Part model, mm, in its own coordinate system. A direction names the side the tool comes from. Give positions to 0.01 mm unless a question says otherwise; leave off trailing zeros. Write each loop counter-clockwise with the first axis right and the second up, starting at its lowest first coordinate (ties: lowest second). Pieces come first, ordered by that corner, then holes.
```python
from build123d import *

# Parameters (mm, degrees)
SALIENTE_EXTRUIR1_DEPTH      = 45
CORTAR_EXTRUIR1_DEPTH        = 35
CORTAR_EXTRUIR1_DEPTH_BACK   = 25
SALIENTE_EXTRUIR2_DEPTH      = 0.0001
SALIENTE_EXTRUIR2_DEPTH_BACK = 10
CORTAR_EXTRUIR2_DEPTH        = 50.0001
CROQUIS5_R                   = 2.5
CORTAR_EXTRUIR3_DEPTH        = 20
CROQUIS6_W                   = 35
CROQUIS6_H                   = 5
CORTAR_EXTRUIR4_DEPTH        = 50
REDONDEO7_R                  = 10
SALIENTE_EXTRUIR3_DEPTH      = 45


with BuildPart() as part:
    # Croquis1 → Saliente-Extruir1 (new body)
    with BuildSketch(Plane.XY):
        with BuildLine():
            Line((5.169872345, 17.452931937), (-42.830127655, 37.452931937))
            Line((-42.830127655, 37.452931937), (-42.830127655, 17.452931937))
            Line((-42.830127655, 17.452931937), (-34.437895384, -24.508229414))
            ThreePointArc((-34.437895384, -24.508229414), (-30.971977683, -30.280489476), (-24.632088627, -32.547068063))
            Line((-24.632088627, -32.547068063), (-22.830127655, -32.547068063))
            Line((-22.830127655, -32.547068063), (-22.830127655, -12.547068063))
            ThreePointArc((-22.830127655, -12.547068063), (-18.830127655, -8.547068063), (-14.830127655, -12.547068063))
            Line((-14.830127655, -12.547068063), (-14.830127655, -32.547068063))
            Line((-14.830127655, -32.547068063), (-13.028166682, -32.547068063))
            ThreePointArc((-13.028166682, -32.547068063), (-6.688277626, -30.280489476), (-3.222359925, -24.508229414))
            Line((-3.222359925, -24.508229414), (5.169872345, 17.452931937))
        make_face()
    extrude(amount=SALIENTE_EXTRUIR1_DEPTH)

    # Croquis2 → Cortar-Extruir1 (cut, two sides: drawn at the far end of the back side and taken through both)
    with BuildSketch(Plane(origin=(-22.830127655, 0, 0), x_dir=(0, 0, -1), z_dir=(1, 0, 0)).offset(-CORTAR_EXTRUIR1_DEPTH_BACK)):
        Polygon((-40, -32.547068063), (-5, -32.547068063), (-5, 11.74295153), (-5, 27.452931937), (-40, 27.382795607), (-40, 11.74295153), align=None)
    extrude(amount=CORTAR_EXTRUIR1_DEPTH + CORTAR_EXTRUIR1_DEPTH_BACK, mode=Mode.SUBTRACT)

    # Croquis3 → Saliente-Extruir2 (add, two sides: drawn at the far end of the back side and taken through both)
    with BuildSketch(Plane(origin=(6.961081212, 16.706594909, 0), x_dir=(0.9230769230769231, -0.38461538461538447, 0), z_dir=(0.38461538461538447, 0.9230769230769231, 0)).offset(-SALIENTE_EXTRUIR2_DEPTH_BACK)):
        Polygon((-53.940476272, -45), (-53.940476272, 0), (-1.940476272, 0), (5.740404043, 0), (5.740404043, -45), (-1.940476272, -45), align=None)
    extrude(amount=SALIENTE_EXTRUIR2_DEPTH + SALIENTE_EXTRUIR2_DEPTH_BACK)

    # Croquis4 → Cortar-Extruir2 (cut)
    with BuildSketch(Plane.XY.offset(45)):
        Polygon((-42.830127655, 17.452931937), (-42.830127655, 41.659540507), (3.169872345, 41.659540507), (3.169872345, 7.452931937), (4.911234771, 4.934595431), (17.135740174, 1.881036512), (16.246125069, 53.47871262), (-56.321049949, 53.47871262), (-56.321049949, 17.452931937), align=None)
    extrude(amount=-CORTAR_EXTRUIR2_DEPTH, mode=Mode.SUBTRACT)

    # Croquis5 → Cortar-Extruir3 (cut)
    with BuildSketch(Plane(origin=(6.961119674, 16.706687217, 0), x_dir=(0.9230769230769231, -0.3846153846153847, 0), z_dir=(0.38461538461538464, 0.923076923076923, 0))):
        with Locations(Location((-29.023830439, -22.5, 0), (0, 0, 180))):
            Circle(CROQUIS5_R)
    extrude(amount=-CORTAR_EXTRUIR3_DEPTH, mode=Mode.SUBTRACT)

    # Croquis6 → Cortar-Extruir4 (cut)
    with BuildSketch(Plane(origin=(3.169872345, 0, 0), x_dir=(0, 0, -1), z_dir=(1, 0, 0))):
        with Locations((-22.5, 9.952931937)):
            Rectangle(CROQUIS6_W, CROQUIS6_H)
    extrude(amount=-CORTAR_EXTRUIR4_DEPTH, mode=Mode.SUBTRACT)

    # Redondeo7
    # the kernel refuses this fillet: 10 mm, written as the material it takes off along each edge
    with BuildSketch(Plane(origin=(3.169872345, 12.452931937, 40), x_dir=(-1, 0, 0), z_dir=(0, 0, -1))) as redondeo7_piece_1:
        with BuildLine():
            CenterArc((REDONDEO7_R, REDONDEO7_R), REDONDEO7_R, 180, 90)
            Line((0, REDONDEO7_R), (0, 0))
            Line((0, 0), (REDONDEO7_R, 0))
        make_face()
    extrude(amount=35, mode=Mode.SUBTRACT)

    # Croquis7 → Saliente-Extruir3 (add)
    with BuildSketch(Plane.XY.offset(45)):
        Polygon((0.400641576, 19.440219758), (1.939103115, 23.13252745), (3.169872345, 18.286373604), align=None)
    extrude(amount=-SALIENTE_EXTRUIR3_DEPTH)


solid = part.part
```
1) Saw through at B-B, the plane y = -26.5. Write the cut outline in (x, z).
Answers follow:
outline: (-33.82, 0) - (-22.83, 0) - (-22.83, 5) - (-33.82, 5) - close; (-33.82, 40) - (-22.83, 40) - (-22.83, 45) - (-33.82, 45) - close; (-14.83, 0) - (-3.84, 0) - (-3.84, 5) - (-14.83, 5) - close; (-14.83, 40) - (-3.84, 40) - (-3.84, 45) - (-14.83, 45) - close
2) Wall check: L1, parallel to Z at x = -14.5, y = 9; L2, parallel to X at y = 20.5, z = 9.5; L3, parallel to Y at x = -33, z = 21. Give the ranges that are in metal, low to high.
Answers follow:
L1: z = 0 to 5, 40 to 45
L2: x = -28.14 to -2.14, 0.84 to 2.61
L3: y = 22.52 to 33.36
3) 3-axis set-ups, long thin cutter, end or side, ignore diameter. For faces 4 (the face through (-22.967, 23.836, 24.608)), 5 (the face through (-22.83, -23, 42)), 6 (the face through (-20.91, 28.32, 17.19)): which of +Z, -Z, +X, -X, +Y, -Y reach the whole face in a straight line?
Answers follow:
face 4: none
face 5: +Z, -Z, -Y
face 6: +Z, -Z, +Y
4) Saw through at C-C, the plane x = -1. Write the cut outline in (y, z).
Answers follow:
outline: (-13.4, 0) - (20.02, 0) - (20.02, 45) - (-13.4, 45) - (-13.4, 40) - (14.33, 40) - (14.33, 5) - (-13.4, 5) - close
5) Two-plate mould, pull along Z, no slides. Class faces 1 (the face through (-20, -3, 5)), 2 (the face through (1.16, 21.26, 22.82)), 3 (the face through (-25.592, 19.437, 26.144)): +Z half, -Z half, draft (parallel to the pull), parting line (faces both ways), or undercut.
Answers follow:
face 1: undercut
face 2: draft
face 3: undercut
6) Pin check, flat tips, straight feed: pin 1 Ø1 at (x, z) = (-8.5, 20.5) entering from -Y; pin 2 Ø5.5 at (y, z) = (-21.5, 43.5) entering from -X; pin 3 Ø1.5 at (x, z) = (-8, 24.5) entering from +Y. Stop position of each tip, or through.
Answers follow:
pin 1: stops at y = 12.45
pin 2: stops at x = -35.59
pin 3: stops at y = 23.25
